from build123d import *

# Parameters (mm, degrees)
BASE_PLATE_DEPTH         = 3
INNER_START              = -3
INNER_BASE_PROFILE_DEPTH = 4
MOUNTING_START           = -7
BASEPLATE_5_R            = 1.65
MOUNTING_HOLES_DEPTH     = 7
COUNTERSINK_SIZE         = 1.7


with BuildPart() as part:
    # BasePlate → Base Plate (new body)
    with BuildSketch(Plane(origin=(0, 0, 0), x_dir=(1, 0, 0), z_dir=(0, 1, 0))):
        with BuildLine():
            Line((-85, 75), (85, 75))
            ThreePointArc((85, 75), (95.606601718, 70.606601718), (100, 60))
            Line((100, 60), (100, -60))
            ThreePointArc((100, -60), (95.606601718, -70.606601718), (85, -75))
            Line((85, -75), (-85, -75))
            ThreePointArc((-85, -75), (-95.606601718, -70.606601718), (-100, -60))
            Line((-100, -60), (-100, 60))
            ThreePointArc((-100, 60), (-95.606601718, 70.606601718), (-85, 75))
        make_face()
    extrude(amount=-BASE_PLATE_DEPTH)

    # BasePlate<4> → Inner Base Profile (add)
    with BuildSketch(Plane(origin=(0, 0, 0), x_dir=(1, 0, 0), z_dir=(0, 1, 0)).offset(INNER_START)):
        with BuildLine():
            Line((-85, 73), (46, 73))
            ThreePointArc((46, 73), (47.414213562, 72.414213562), (48, 71))
            ThreePointArc((48, 71), (50, 69), (52, 71))
            ThreePointArc((52, 71), (52.585786438, 72.414213562), (54, 73))
            Line((54, 73), (85, 73))
            ThreePointArc((85, 73), (94.192388155, 69.192388155), (98, 60))
            Line((98, 60), (98, -60))
            ThreePointArc((98, -60), (94.192388155, -69.192388155), (85, -73))
            Line((85, -73), (54, -73))
            ThreePointArc((54, -73), (52.585786438, -72.414213562), (52, -71))
            ThreePointArc((52, -71), (50, -69), (48, -71))
            ThreePointArc((48, -71), (47.414213562, -72.414213562), (46, -73))
            Line((46, -73), (-85, -73))
            ThreePointArc((-85, -73), (-94.192388155, -69.192388155), (-98, -60))
            Line((-98, -60), (-98, 60))
            ThreePointArc((-98, 60), (-94.192388155, 69.192388155), (-85, 73))
        make_face()
    extrude(amount=-INNER_BASE_PROFILE_DEPTH)

    # BasePlate<5> → Mounting Holes (cut)
    with BuildSketch(Plane(origin=(0, 0, 0), x_dir=(1, 0, 0), z_dir=(0, 1, 0)).offset(MOUNTING_START)):
        with Locations(Location((90, -15, 0), (0, 0, 270))):
            Circle(BASEPLATE_5_R)
        with Locations(Location((-89, 64, 0), (0, 0, 270))):
            Circle(BASEPLATE_5_R)
        with Locations(Location((89, 64, 0), (0, 0, 270))):
            Circle(BASEPLATE_5_R)
        with Locations(Location((89, -64, 0), (0, 0, 270))):
            Circle(BASEPLATE_5_R)
        with Locations(Location((-89, -64, 0), (0, 0, 270))):
            Circle(BASEPLATE_5_R)
        with Locations(Location((0, 65, 0), (0, 0, 270))):
            Circle(BASEPLATE_5_R)
        with Locations(Location((-90, 0, 0), (0, 0, 270))):
            Circle(BASEPLATE_5_R)
        with Locations(Location((0, -65, 0), (0, 0, 270))):
            Circle(BASEPLATE_5_R)
    extrude(amount=MOUNTING_HOLES_DEPTH, mode=Mode.SUBTRACT)

    # Countersink
    countersink_edges = [part.edges().sort_by_distance(p)[0] for p in [
        (-89, 0, 62.35),
        (0, 0, -66.65),
        (89, 0, -65.65),
        (90, 0, 13.35),
        (89, 0, 62.35),
        (-90, 0, -1.65),
        (-89, 0, -65.65),
        (0, 0, 63.35),
    ]]
    chamfer(countersink_edges, length=COUNTERSINK_SIZE)


solid = part.part
Model file for the job. Use its own axes, mm. A direction names the side the tool comes from. Round coordinates to 2 decimals unless told otherwise and drop trailing zeros. Loops run counter-clockwise (first coordinate to the right, second up) from the corner with the lowest first, then second, coordinate; pieces in that order, holes last.
1. Band-saw the part on A-A, the plane x = -57. List the corners of the cut face in (y, z).
Check values:
outline: (-7, -73) - (-3, -73) - (-3, -75) - (0, -75) - (0, 75) - (-3, 75) - (-3, 73) - (-7, 73) - close
2. Wall check: probe 1 along Z at (x, y) = (89, -5.85); probe 2 along X at (y, z) = (-4.25, -64); probe 3 along Z at (x, y) = (-88, -3.25). Give the ranges that are in metal, low to high.
Check values:
probe 1: z = -72.37 to -65.65, -62.35 to 13.69, 16.31 to 62.35, 65.65 to 72.37
probe 2: x = -97.37 to -90.65, -87.35 to -1.31, 1.31 to 87.35, 90.65 to 97.37
probe 3: z = -72.65 to -65.31, -62.69 to 62.69, 65.31 to 72.65
3. Drop flat-ended pins along their axis: P1, Ø4.5, axis at x = -89, z = -64, coming from the +Y side; P2, Ø5.5, axis at x = 89, z = 64, coming from the +Y side; P3, Ø5.5, axis at x = -89, z = 64, coming from the -Y side; P4, Ø3, axis at x = 64.5, y = -5, coming from the -Z side. Give the stop position or say it passes through.
Check values:
P1: stops at y = -1.1
P2: stops at y = -0.6
P3: stops at y = -7
P4: stops at z = -73
4. Tool access for faces 1 (the cylindrical face through (-94.293, -4.972, -69.091)), 2 (the flat face through (-98, -5, 1)), 3 (the cylindrical face through (94.091, -4.972, -69.293)): list every direction of +Z, -Z, +X, -X, +Y, -Y with a clear straight run to the whole face (end or side of a thin tool).
Check values:
face 1: -Z, -X, -Y
face 2: +Z, -Z, -X, -Y
face 3: -Z, +X, -Y
